Here's how the part is built. I have some questions about the finished solid (model axes, mm). Round coordinates to 2 decimals unless told otherwise and drop trailing zeros. Loops run counter-clockwise (first coordinate to the right, second up) from the corner with the lowest first, then second, coordinate; pieces in that order, holes last. Notation, with made-up numbers: M 40,82 L 95,82 A5 cw 95,88 Z; hole C 83.25,-3 d6. An arc over 180 degrees is marked long. Answer as a JSON object with one key per item and string values.
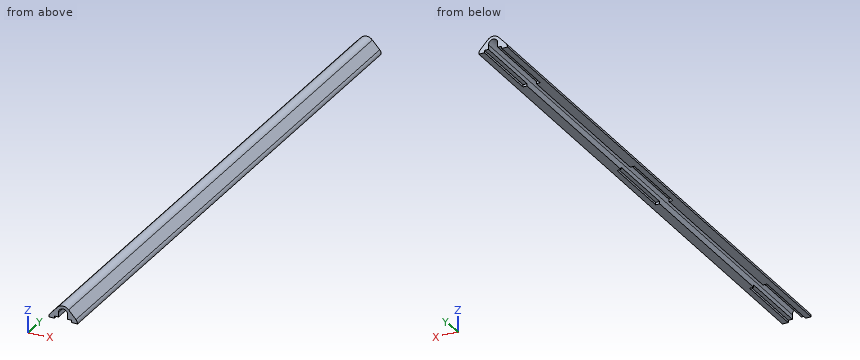
Autodesk Fusion 360 part; units mm, degrees
sketch "Sketch1" plane through (0, 0, 0) normal (0, 1, 0) x (1, 0, 0) in component "Main"
  arc A0 (-1.9148, -3.3588) -> (1.9148, -3.3588) centre (0, -1.6) ccw
  line L0 (-1.9148, -3.3588) -> (-5, 0)
  line L1 (1.9148, -3.3588) -> (5, 0)
  line L2 (-5, 0) -> (5, 0)
  line L3 (0, -1.6) -> (0, 0) construction
  circle A1 centre (0, -1.6) radius 1.5 construction
  arc A2 (-1.6, -1.6) -> (1.6, -1.6) centre (0, -1.6) ccw
  line L4 (-1.6, -1.6) -> (-1.6, 0)
  line L5 (1.6, -1.6) -> (1.6, 0)
  point P0 (0, -0.1)
  dimension "d3" = 0.1
  dimension "d4" = 3
  dimension "d5" = 0.1
  dimension "d6" = 1
  dimension "d7" = 85.137
  dimension "d12" = 10
extrude "Extrude1" add sketch "Sketch1" along normal mid plane 200 contours A0 L0 L1 L2 A2 L4 L5 in component "Main"
sketch "Sketch2" plane through (0, 0, 0) normal (0, 0, 1) x (1, 0, 0) in component "Main"
  line L0 (-5, -100) -> (-5, 100)
  line L1 (5, -100) -> (5, 100)
  line L2 (3, -100) -> (-3, -100)
  line L3 (-3, -100) -> (-3, -74.6)
  line L4 (-3, -74.6) -> (3, -74.6)
  line L5 (3, -74.6) -> (3, -100)
  line L6 (-5, -100) -> (3, -74.6) construction
  line L7 (5, -100) -> (-3, -74.6) construction
  line L8 (3, 100) -> (-3, 100)
  line L9 (-3, 100) -> (-3, 74.6)
  line L10 (-3, 74.6) -> (3, 74.6)
  line L11 (3, 74.6) -> (3, 100)
  line L12 (3, -12.7) -> (-3, -12.7)
  line L13 (-3, -12.7) -> (-3, 12.7)
  line L14 (-3, 12.7) -> (3, 12.7)
  line L15 (3, 12.7) -> (3, -12.7)
  line L16 (3, 0) -> (-3, 0) construction
  line L17 (-5, -100) -> (-3, -100)
  line L18 (5, -100) -> (3, -100)
  line L19 (5, 100) -> (3, 100)
  line L20 (-3, 100) -> (-5, 100)
  line L21 (1.6, -100) -> (1.6, 100)
  line L22 (-1.6, -100) -> (-1.6, 100)
  dimension "d17" = 25.4
  dimension "d18" = 2
  dimension "d19" = 25.4
  dimension "d20" = 25.4
extrude "Extrude2" add sketch "Sketch2" against normal blind 0.8 contours L0 L3 L4 L9 L10 L12 L13 L14 L17 L20 L22 | L1 L4 L5 L10 L11 L12 L14 L15 L18 L19 L21 in component "Main"
sketch "Sketch3" plane through (0, 0, 0) normal (0, 1, 0) x (1, 0, 0) in component "Main"
  line L0 (-5, 0) -> (-1.9148, -3.3588)
  line L1 (-5, 0.8) -> (-5, 0)
  arc A0 (-5, 0.8) -> (-4.4588, -0.5892) centre (-2.9464, 0.8) ccw
  line L2 (-5, 0.8) -> (-3, 0.8)
  dimension "d23" = 2.0536
fillet "Fillet1" radius 2.0536 2 edges at (-5, 0, 0) (5, 0, 0) in component "Main"
split "Split1" [suppressed] in component "Main"
extrude "Extrude3" [suppressed] in component "Main"
component "Main" placed x (1, 0, 0) y (0, 1, 0) z (0, 0, 1) at (0, 0, 0)
equation "d4 = CableDiameter"
equation "CableDiameter = 3 mm"
equation "BotWidth = 10 mm"
equation "d12 = BotWidth"
equation "GapWidth = 25.4 mm"
equation "d17 = GapWidth"
equation "d19 = GapWidth"
equation "d20 = GapWidth"
equation "d25 = d23"
Item 1: Please list where these lines run through material, in increasing order: probe 1 along Z at (x, y) = (3.5, 40); probe 2 along X at (y, z) = (28, 1.4); probe 3 along X at (y, z) = (-14.5, 0.6). Write a range as from..to.
Resolved:
{"probe 1": "-0.8..1.63", "probe 2": "-3.71..-1.6, 1.6..3.71", "probe 3": "-4.45..-1.6, 1.6..4.45"}
Item 2: I'm going to push flat-ended pins straight in: pin 1 Ø1.5 at (x, y) = (-2, 4) entering from -Z; pin 2 Ø0.6 at (x, z) = (2.5, -0.5) entering from -Y; pin 3 Ø2 at (x, y) = (-3, -18.5) entering from +Z. Where does each tip first touch, or does it pass through?
Resolved:
{"pin 1": "z = 0", "pin 2": "y = -74.6", "pin 3": "z = 3.27"}
Item 3: I want a section at B-B, the plane z = 2.4. Please give me the cut outline in (x, y).
Resolved:
{"outline": "M -2.8,-100 L -1.39,-100 L -1.39,100 L -2.8,100 Z; M 1.39,-100 L 2.8,-100 L 2.8,100 L 1.39,100 Z"}
Item 4: I want a section at C-C, the plane x = 0. Please give me the cut outline in (y, z), then the cut area to 3 significant figures.
Resolved:
{"outline": "M -100,3.2 L 100,3.2 L 100,4.2 L -100,4.2 Z", "area": "200 mm²"}
